Input: dimensioned drawing with shaded views. Units: mm. Origin: part minimum x, y, z. A direction names the side the tool comes from. Coordinates: 2 decimals unless noted, no trailing zeros. Order: outer loops, then holes, each group sorted by start corner. A loop starts at its lowest first (then second) coordinate and runs counter-clockwise, first axis right, second up. Notation, with made-up numbers: (24, 89.5) - (80, 89.5) arc R12 cw to (80, 93.5) - close; hole circle Ø4 at (44.25, 84.5). An arc over 180 degrees is marked (long way). One line per question, with ' | ' between items. Start each with the question number.
(1) Access query for the marked faces 1 and 2. Directions: +Z, -Z, +X, -X, +Y, -Y. A direction counts if a zero-diameter tool reaches every point of the face in a straight line with its end or side. Return the directions, or none.
(2) Section A-A (y = 33.5). Return the cut outline in (x, z), then the cut area to 3 significant figures.
(3) Section C-C (y = 25.4). Return the cut outline in (x, z) (3 decimals).
(4) Line query: line 1 along X through (y, z) = (24.5, 3.25); line 2 along X through (y, z) = (28, 1.75); line 3 along Y through (x, z) = (38.1, 3). Output: solid intervals per line, ascending.
(5) Section D-D (z = 4.5). Count the separate pieces of the cut face and the enclosed holes in it, then the cut area to 3 significant figures.
(6) Section B-B (x = 17). Return the cut outline in (y, z).
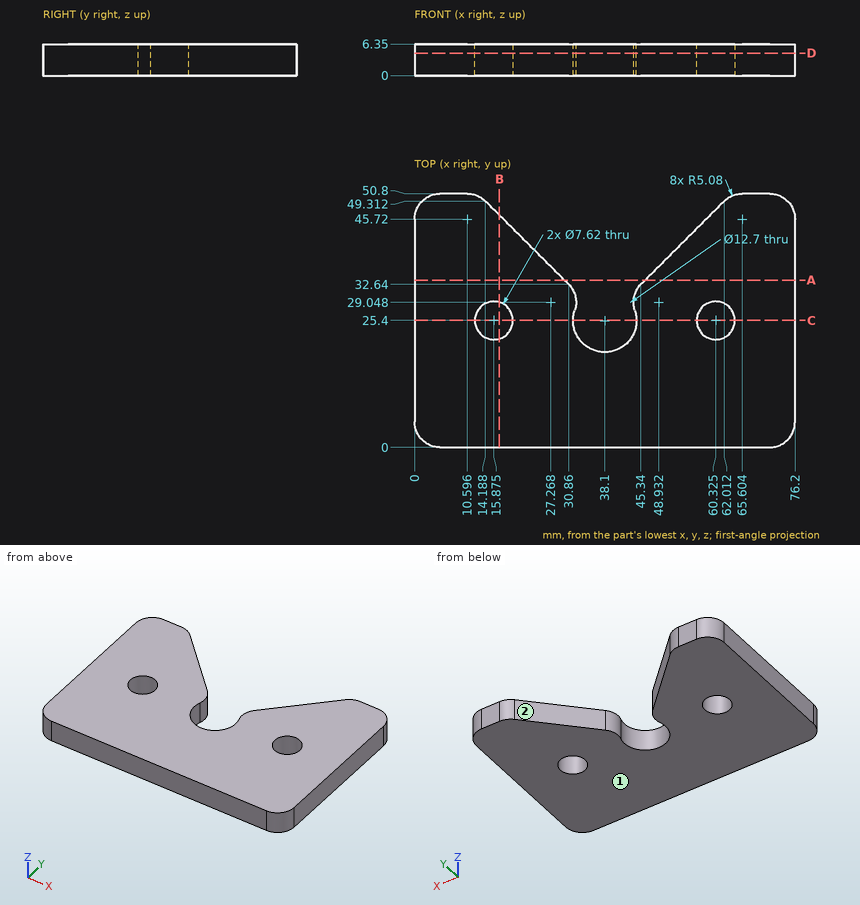
Response values:
1) face 1: -Z, +X, -X, +Y, -Y | face 2: +Z, -Z, +Y
2) outline: (0, 0) - (30, 0) - (30, 6.35) - (0, 6.35) - close; (46.2, 0) - (76.2, 0) - (76.2, 6.35) - (46.2, 6.35) - close | area: 381 mm²
3) outline: (0, 0) - (12.065, 0) - (12.065, 6.35) - (0, 6.35) - close; (19.685, 0) - (31.75, 0) - (31.75, 6.35) - (19.685, 6.35) - close; (44.45, 0) - (56.515, 0) - (56.515, 6.35) - (44.45, 6.35) - close; (64.135, 0) - (76.2, 0) - (76.2, 6.35) - (64.135, 6.35) - close
4) line 1: x = 0 to 12.17, 19.58 to 31.81, 44.39 to 56.62, 64.03 to 76.2 | line 2: x = 0 to 13.09, 18.66 to 32.24, 43.96 to 57.54, 63.11 to 76.2 | line 3: y = 0 to 19.05
5) separate pieces: 1 | enclosed holes: 2 | area: 3,010 mm²
6) outline: (0, 0) - (21.76, 0) - (21.76, 6.35) - (0, 6.35) - close; (29.04, 0) - (46.5, 0) - (46.5, 6.35) - (29.04, 6.35) - close
